```python
from build123d import *

# Parameters (mm, degrees)
F1_DEPTH = 25.4


with BuildPart() as f1:
    # F0 (on Right) → F1 (new body)
    with BuildSketch(Plane.YZ):
        with BuildLine():
            Line((228.6, 376.9212961197), (0, 376.9212961197))
            Line((0, 376.9212961197), (-228.6, 376.9212961197))
            add(Edge.make_bspline(
                [(-457.2753436089, 347.454816103), (-428.9132900906, 355.8432406544), (-365.8930365544, 374.4822521654), (-277.3142184262, 376.0558762636), (-228.6, 376.9212961197)],
                knots=[0, 0, 0, 0, 0.4500466426, 1, 1, 1, 1], degree=3))
            ThreePointArc((-457.2753436089, 347.454816103), (-551.68686479, 185.9850935796), (-571.5753436089, 0))
            Line((-571.5753436089, 0), (0, 0))
            Line((0, 0), (571.5753436089, 0))
            ThreePointArc((571.5753436089, 0), (551.68686479, 185.9850935796), (457.2753436089, 347.454816103))
            add(Edge.make_bspline(
                [(457.2753436089, 347.454816103), (428.9132900906, 355.8432406544), (365.8930365544, 374.4822521654), (277.3142184262, 376.0558762636), (228.6, 376.9212961197)],
                knots=[0, 0, 0, 0, 0.4500466426, 1, 1, 1, 1], degree=3))
        make_face()
    extrude(amount=F1_DEPTH)


solid = f1.part
```
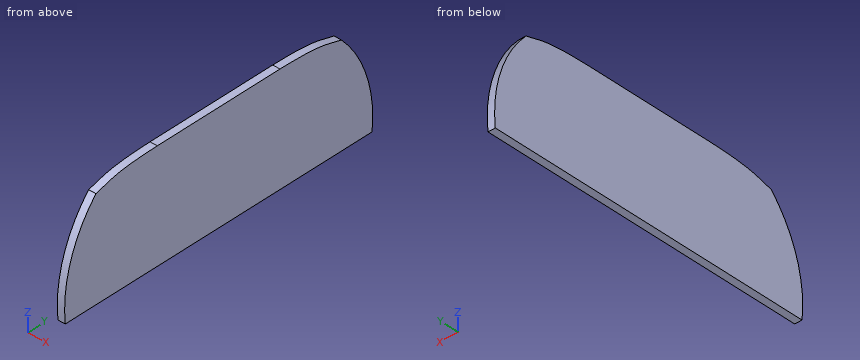
Model file for the job. Use its own axes, mm. Coordinates: 2 decimals unless noted, no trailing zeros. Order: outer loops, then holes, each group sorted by start corner. A loop starts at its lowest first (then second) coordinate and runs counter-clockwise, first axis right, second up. Notation, with made-up numbers: M 32,-3.75 L 47,-3.75 A26 ccw 47,35.25 Z; hole C 44,27 d4. An arc over 180 degrees is marked long. Answer as CSV lines item,"result".
(1) Wall check: line 1 along Y through (x, z) = (8.25, 34); line 2 along Y through (x, z) = (13, 53.5); line 3 along Z through (x, y) = (7.5, 516). Give the ranges that are in metal, low to high.
Geometry says:
line 1,"y = -573.84 to 573.84"
line 2,"y = -573.97 to 573.97"
line 3,"z = 0 to 266.59"
(2) Flat gauge pins, fed straight in: pin 1 (4 mm diameter, centred on x = 16, z = 217.5, fed in from -Y); pin 2 (3 mm diameter, centred on x = 9.5, z = 208.5, fed in from -Y); pin 3 (2 mm diameter, centred on x = 20, z = 93, fed in from -Y). Where does each tip first touch, or does it go through?
Geometry says:
pin 1,"stops at y = -540.81"
pin 2,"stops at y = -544.19"
pin 3,"stops at y = -571.71"
(3) Band-saw the part on B-B, the plane z = 292.5. List the corners of the cut face in (x, y).
Geometry says:
outline,"M 0,-500.12 L 25.4,-500.12 L 25.4,500.12 L 0,500.12 Z"
(4) Band-saw the part on A-A, the plane z = 205.5. List the corners of the cut face in (x, y), then the cut area to 3 significant figures.
Geometry says:
outline,"M 0,-544.76 L 25.4,-544.76 L 25.4,544.76 L 0,544.76 Z"
area,"27,700 mm2"
